Read the model definition and answer for the solid it produces. Units are mm, in the model's axes. Give positions to 0.01 mm unless a question says otherwise; leave off trailing zeros. Loops run counter-clockwise (first coordinate to the right, second up) from the corner with the lowest first, then second, coordinate; pieces in that order, holes last. Notation, with made-up numbers: M 1,77 L 46,77 A10 ccw 46,82 Z; hole C -2.5,75.5 d9. An arc over 180 degrees is marked long. Return JSON: item names as keys, results as strings. Group by question number.
```python
from build123d import *

# Parameters (mm, degrees)
SKETCH_R        = 16.5
PAD_DEPTH       = 13
SKETCH002_R     = 3.25
POCKET_DEPTH    = 13.001
SKETCH001_R     = 5.5
POCKET001_DEPTH = 5
CHAMFER_SIZE    = 1
CHAMFER001_SIZE = 1
CHAMFER002_SIZE = 1


with BuildPart() as part:
    # Sketch → Pad (new body)
    with BuildSketch(Plane.XY):
        Circle(SKETCH_R)
    extrude(amount=PAD_DEPTH)

    # Sketch002 (on Face3 of Pad) → Pocket (cut, through all)
    with BuildSketch(Plane.XY.offset(13)):
        Circle(SKETCH002_R)
    extrude(amount=-POCKET_DEPTH, mode=Mode.SUBTRACT)

    # Sketch001 (on Face3 of Pad) → Pocket001 (cut)
    with BuildSketch(Plane.XY.offset(13)):
        Circle(SKETCH001_R)
    extrude(amount=-POCKET001_DEPTH, mode=Mode.SUBTRACT)

    # Chamfer
    chamfer_edges = [part.edges().sort_by_distance(p)[0] for p in [
        (-16.5, 0, 0),
    ]]
    chamfer(chamfer_edges, length=CHAMFER_SIZE)

    # Chamfer001
    chamfer001_edges = [part.edges().sort_by_distance(p)[0] for p in [
        (-16.5, 0, 13),
    ]]
    chamfer(chamfer001_edges, length=CHAMFER001_SIZE)

    # Chamfer002
    chamfer002_edges = [part.edges().sort_by_distance(p)[0] for p in [
        (-5.5, 0, 13),
    ]]
    chamfer(chamfer002_edges, length=CHAMFER002_SIZE)


solid = part.part
```
1. Find section B-B (z = 5.5). Write down the section's boundary in (x, y), and give its area (3 significant figures).
2. The mould has two halves that part along Y. Classify faces 1 (the cylindrical face through (15.24, -6.32, 6.42)), 2 (the flat face through (4, 0, 8)), 3 (the cylindrical face through (-1.19, -5.37, 10.03)), 4 (the flat face through (7, 0, 13)): +Y half, -Y half, draft (parallel to the pull), parting line (faces both ways), or undercut.
3. Find section C-C (z = 10). Write down the section's boundary in (x, y), and give its area (3 significant figures).
4. Find section A-A (y = 0). Write down the section's boundary in (x, z), and give its area (3 significant figures).
5. Flat-ended cylindrical pins translate along their axes: P1, Ø1, axis at x = -3.5, y = -4, coming from the +Z side; P2, Ø3.5, axis at x = -2.5, y = -2.5, coming from the +Z side; P3, Ø1, axis at x = -1, z = 11.5, coming from the -Y side; P4, Ø6, axis at x = 0, y = 0, coming from the +Z side. Find the tip coordinate at first contact, or state that the pin passes through.
6. Straight lines are drawn through the part: line 1 along Y through (x, z) = (0, 10.85); line 2 along Y through (x, z) = (0, 5.75); line 3 along Z through (x, y) = (2, -4). For each, find the intervals that lie inside material, in ascending order.
Result:
{
 "1": {"outline": "C 0,0 d33; hole C 0,0 d6.5", "area": "822 mm2"},
 "2": {"face 1": "parting line", "face 2": "undercut", "face 3": "undercut", "face 4": "draft"},
 "3": {"outline": "C 0,0 d33; hole C 0,0 d11", "area": "760 mm2"},
 "4": {"outline": "M -16.5,1 L -15.5,0 L -3.25,0 L -3.25,8 L -5.5,8 L -5.5,12 L -6.5,13 L -15.5,13 L -16.5,12 Z; M 3.25,0 L 15.5,0 L 16.5,1 L 16.5,12 L 15.5,13 L 6.5,13 L 5.5,12 L 5.5,8 L 3.25,8 Z", "area": "319 mm2"},
 "5": {"P1": "stops at z = 12.32", "P2": "stops at z = 8", "P3": "stops at y = -16.49", "P4": "passes through"},
 "6": {"line 1": "y = -16.5 to -5.5, 5.5 to 16.5", "line 2": "y = -16.5 to -3.25, 3.25 to 16.5", "line 3": "z = 0 to 8"}
}
